from build123d import *

# Parameters (mm, degrees)
F1_DEPTH = 500


with BuildPart() as f1:
    # F0 (on Top) → F1 (new body)
    with BuildSketch(Plane.XY):
        with BuildLine():
            Line((-30, 50), (-50, 50))
            Line((-50, 50), (-50, 30))
            Line((-50, 30), (-44, 30))
            Line((-44, 30), (-44, 35))
            Line((-44, 35), (-37, 35))
            Line((-37, 35), (-37, 25.5))
            Line((-37, 25.5), (-30.97913, 25.5))
            ThreePointArc((-30.97913, 25.5), (-29.242641, 29.242641), (-25.5, 30.97913))
            ThreePointArc((-25.5, 30.97913), (-20.408156, 28.861991), (-19.195037, 23.482633))
            Line((-19.195037, 23.482633), (-12.5, 30.17767))
            Line((-12.5, 30.17767), (12.5, 30.17767))
            Line((12.5, 30.17767), (19.195037, 23.482633))
            ThreePointArc((19.195037, 23.482633), (29.242641, 29.242641), (23.482633, 19.195037))
            Line((23.482633, 19.195037), (30.17767, 12.5))
            Line((30.17767, 12.5), (30.17767, -12.5))
            Line((30.17767, -12.5), (23.482633, -19.195037))
            ThreePointArc((23.482633, -19.195037), (29.242641, -29.242641), (19.195037, -23.482633))
            Line((19.195037, -23.482633), (12.5, -30.17767))
            Line((12.5, -30.17767), (-12.5, -30.17767))
            Line((-12.5, -30.17767), (-19.195037, -23.482633))
            ThreePointArc((-19.195037, -23.482633), (-29.242641, -29.242641), (-23.482633, -19.195037))
            Line((-23.482633, -19.195037), (-30.17767, -12.5))
            Line((-30.17767, -12.5), (-30.17767, 12.5))
            Line((-30.17767, 12.5), (-23.482633, 19.195037))
            ThreePointArc((-23.482633, 19.195037), (-28.465904, 20.102295), (-30.97913, 24.5))
            Line((-30.97913, 24.5), (-37, 24.5))
            Line((-37, 24.5), (-37, 15))
            Line((-37, 15), (-44, 15))
            Line((-44, 15), (-44, 20))
            Line((-44, 20), (-50, 20))
            Line((-50, 20), (-50, -20))
            Line((-50, -20), (-44, -20))
            Line((-44, -20), (-44, -15))
            Line((-44, -15), (-37, -15))
            Line((-37, -15), (-37, -35))
            Line((-37, -35), (-44, -35))
            Line((-44, -35), (-44, -30))
            Line((-44, -30), (-50, -30))
            Line((-50, -30), (-50, -50))
            Line((-50, -50), (-30, -50))
            Line((-30, -50), (-30, -44))
            Line((-30, -44), (-35, -44))
            Line((-35, -44), (-35, -37))
            Line((-35, -37), (-15, -37))
            Line((-15, -37), (-15, -44))
            Line((-15, -44), (-20, -44))
            Line((-20, -44), (-20, -50))
            Line((-20, -50), (20, -50))
            Line((20, -50), (20, -44))
            Line((20, -44), (15, -44))
            Line((15, -44), (15, -37))
            Line((15, -37), (35, -37))
            Line((35, -37), (35, -44))
            Line((35, -44), (30, -44))
            Line((30, -44), (30, -50))
            Line((30, -50), (50, -50))
            Line((50, -50), (50, -30))
            Line((50, -30), (44, -30))
            Line((44, -30), (44, -35))
            Line((44, -35), (37, -35))
            Line((37, -35), (37, -15))
            Line((37, -15), (44, -15))
            Line((44, -15), (44, -20))
            Line((44, -20), (50, -20))
            Line((50, -20), (50, 20))
            Line((50, 20), (44, 20))
            Line((44, 20), (44, 15))
            Line((44, 15), (37, 15))
            Line((37, 15), (37, 35))
            Line((37, 35), (44, 35))
            Line((44, 35), (44, 30))
            Line((44, 30), (50, 30))
            Line((50, 30), (50, 50))
            Line((50, 50), (30, 50))
            Line((30, 50), (30, 44))
            Line((30, 44), (35, 44))
            Line((35, 44), (35, 37))
            Line((35, 37), (15, 37))
            Line((15, 37), (15, 44))
            Line((15, 44), (20, 44))
            Line((20, 44), (20, 50))
            Line((20, 50), (-20, 50))
            Line((-20, 50), (-20, 44))
            Line((-20, 44), (-15, 44))
            Line((-15, 44), (-15, 37))
            Line((-15, 37), (-25.5, 37))
            Line((-25.5, 37), (-35, 37))
            Line((-35, 37), (-35, 44))
            Line((-35, 44), (-30, 44))
            Line((-30, 44), (-30, 50))
        make_face()
    extrude(amount=F1_DEPTH)


solid = f1.part
Design review of the part built by this model. Coordinates are the model's own, in mm. A direction names the side the tool comes from. Round coordinates to 2 decimals unless told otherwise and drop trailing zeros. Write each loop counter-clockwise with the first axis right and the second up, starting at its lowest first coordinate (ties: lowest second). Pieces come first, ordered by that corner, then holes.
Item 1: Consider section A-A on x = -4. Give the boundary of the cut face in (y, z).
Item 2: Wall thickness on L1, parallel to X at y = -33, z = 130.5; L2, parallel to Y at x = -25, z = 145: over which ranges is each line inside the solid? List them lowest first.
Item 3: For faces 1 (the flat face through (25, 37, 246)), 2 (the flat face through (-34, 1, 500)), list the 3-axis set-ups (+Z, -Z, +X, -X, +Y, -Y) from which the entire face can be reached by the end or side of a thin tool; tool diameter is ignored.
Item 4: Draft analysis for pull direction Y (two halves, no side actions). For faces 3 (the flat face through (40, 50, 246)), 4 (the flat face through (-50, -40, 246)), 5 (the flat face through (37, 25, 246)), state which applies: released by +Y, released by -Y, zero draft, split by the parting line, or undercut.
Item 5: For pin 1 Ø1 at (x, z) = (24, 439.5) entering from +Y; pin 2 Ø5 at (x, y) = (22.5, -24) entering from -Z, all flat-tipped, find the tip position at first contact; note any pin that passes through.
Check values:
1. outline: (-50, 0) - (-30.18, 0) - (-30.18, 500) - (-50, 500) - close; (30.18, 0) - (50, 0) - (50, 500) - (30.18, 500) - close
2. L1: x = -50 to -44, -37 to 37, 44 to 50
2. L2: y = -37 to -31, -19 to -17.68, 17.68 to 19, 31 to 37
3. face 1: +Z, -Z
3. face 2: +Z, +X, -X, +Y, -Y
4. face 3: released by +Y
4. face 4: zero draft
4. face 5: undercut
5. pin 1: stops at y = 37
5. pin 2: passes through
